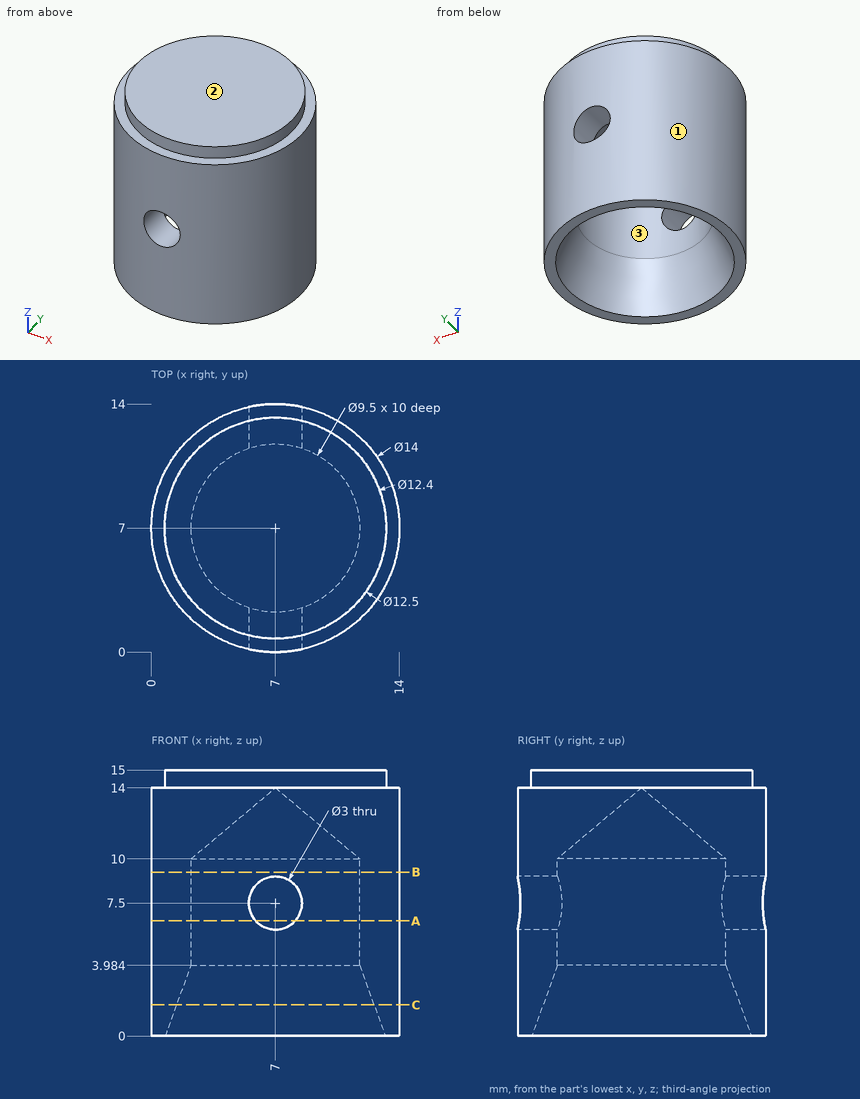
Part print with two shaded views. Sizes in mm from the minimum x, y, z corner. Round coordinates to 2 decimals unless told otherwise and drop trailing zeros. Order: outer loops, then holes, each group sorted by start corner. A loop starts at its lowest first (then second) coordinate and runs counter-clockwise, first axis right, second up. Notation, with made-up numbers: (54.5, 58.5) - (79.5, 58.5) arc R22 ccw to (79.5, 79.5) - close; hole circle Ø1 at (73.5, -34.75). An arc over 180 degrees is marked (long way). Answer in a Markdown table with one row per item. Add a question column.
(1) Band-saw the part on B-B on z = 9.25. List the corners of the cut face in (x, y).
(2) Mould opens along Y. For the marked faces 1, 2 and 3 say: +Y half, -Y half, draft (parallel to the pull), parting line (faces both ways), or undercut.
(3) Drop flat-ended pins along their axis: pin 1 Ø1.8 at (x, z) = (7, 7.5) entering from +Y; pin 2 Ø1.5 at (y, z) = (5, 3) entering from +X; pin 3 Ø4 at (x, z) = (4, 10.5) entering from -Y. Give the stop position or say it passes through.
(4) Band-saw the part on A-A on z = 6.5. List the corners of the cut face in (x, y).
(5) Probe L1, parallel to X at y = 6.75, z = 7.5; L2, parallel to Y at x = 5.5, z = 3.5. List the from-to ranges inside material, lowest first. Write a range as [from, to].
(6) Band-saw the part on C-C on z = 1.75. List the corners of the cut face in (x, y).
Data:
| question | item | result |
|---|---|---|
| 1 | outline | circle Ø14 at (7, 7); hole circle Ø9.5 at (7, 7) |
| 2 | face 1 | parting line |
| 2 | face 2 | draft |
| 2 | face 3 | undercut |
| 3 | pin 1 | passes through |
| 3 | pin 2 | stops at x = 13.89 |
| 3 | pin 3 | stops at y = 0.07 |
| 4 | outline | (5.88, 0.09) - (5.88, 2.38) arc R4.75 cw to (5.88, 11.62) - (5.88, 13.91) arc R7 ccw to start; (8.12, 0.09) arc R7 ccw to (8.12, 13.91) - (8.12, 11.62) arc R4.75 cw to (8.12, 2.38) - close |
| 5 | L1 | x = [0, 2.26], [11.74, 14] |
| 5 | L2 | y = [0.16, 2.31], [11.69, 13.84] |
| 6 | outline | circle Ø14 at (7, 7); hole circle Ø11.13 at (7, 7) |
